from build123d import *

# Parameters (mm, degrees)
SKETCH2_W           = 21
SKETCH2_H           = 21
BOSS_EXTRUDE1_DEPTH = 20
SKETCH3_W           = 15
SKETCH3_H           = 15
CUT_EXTRUDE1_DEPTH  = 20
SKETCH4_W           = 4
SKETCH4_H           = 7.5
BOSS_EXTRUDE2_DEPTH = 20
FILLET2_R           = 2
SKETCH5_W           = 7
SKETCH5_H           = 56
BOSS_EXTRUDE3_DEPTH = 4
SKETCH6_W           = 3
SKETCH6_H           = 56
BOSS_EXTRUDE4_DEPTH = 85
SKETCH8_R           = 1.375
CUT_EXTRUDE2_DEPTH  = 4


with BuildPart() as part:
    # Sketch2 → Boss-Extrude1 (new body)
    with BuildSketch(Plane.XY):
        Rectangle(SKETCH2_W, SKETCH2_H)
    extrude(amount=BOSS_EXTRUDE1_DEPTH)

    # Sketch3 → Cut-Extrude1 (cut)
    with BuildSketch(Plane.XY.offset(20)):
        Rectangle(SKETCH3_W, SKETCH3_H)
    extrude(amount=-CUT_EXTRUDE1_DEPTH, mode=Mode.SUBTRACT)

    # Sketch4 → Boss-Extrude2 (add)
    with BuildSketch(Plane.ZY.offset(10.5)):
        with Locations((2, 0)):
            Rectangle(SKETCH4_W, SKETCH4_H)
    extrude(amount=BOSS_EXTRUDE2_DEPTH)

    # Fillet2
    fillet2_edges = [part.edges().sort_by_distance(p)[0] for p in [
        (-20.5, -3.75, 4),
        (-20.5, 3.75, 4),
    ]]
    fillet(fillet2_edges, radius=FILLET2_R)

    # Sketch5 → Boss-Extrude3 (add)
    with BuildSketch(Plane.ZY.offset(30.5)):
        with Locations((3.5, 0)):
            Rectangle(SKETCH5_W, SKETCH5_H)
    extrude(amount=BOSS_EXTRUDE3_DEPTH)

    # Sketch6 → Boss-Extrude4 (add)
    with BuildSketch(Plane.ZY.offset(34.5)):
        with Locations((1.5, 0)):
            Rectangle(SKETCH6_W, SKETCH6_H)
    extrude(amount=BOSS_EXTRUDE4_DEPTH)

    # Sketch8 → Cut-Extrude2 (cut)
    with BuildSketch(Plane.XY.offset(3)):
        with Locations((-39, -24.5)):
            Circle(SKETCH8_R)
        with Locations((-39, 24.5)):
            Circle(SKETCH8_R)
        with Locations((-97, -24.5)):
            Circle(SKETCH8_R)
        with Locations((-97, 24.5)):
            Circle(SKETCH8_R)
    extrude(amount=-CUT_EXTRUDE2_DEPTH, mode=Mode.SUBTRACT)


solid = part.part
Geometry: final body of the model. Coordinates: model frame, mm. A direction names the side the tool comes from. Coordinates: 2 decimals unless noted, no trailing zeros. Order: outer loops, then holes, each group sorted by start corner. A loop starts at its lowest first (then second) coordinate and runs counter-clockwise, first axis right, second up.
(1) Draft query along X for faces 1 (the face through (0, -10.5, 10)), 2 (the face through (-119.5, 0, 1)), 3 (the face through (-40.013, 25.429, 1.521)). Return one class per face: pulls with the +X half, pulls with the -X half, needs draft (parallel to the pull), parting line crosses it, or undercut.
(2) Section query D-D (x = -25). Return the cut outline in (y, z).
(3) Section query C-C (y = 15.5). Return the cut outline in (x, z), plus the area to 3 significant figures.
(4) First-contact query: pin 1 (4.5 mm diameter, centred on x = 1.5, z = 5.5, fed in from -Y); pin 2 (3 mm diameter, centred on x = -37.5, z = 7.5, fed in from +Y); pin 3 (8 mm diameter, centred on y = 14, z = 13.5, fed in from -X); pin 4 (3 mm diameter, centred on y = 1.5, z = 5.5, fed in from -X). Flat tips, straight axial feed; report the tip coordinate or a pass-through.
(5) Access query for faces 4 (the face through (-20, 0, 4)), 5 (the face through (0, 7.5, 10)), 6 (the face through (-32, 0, 7)), 7 (the face through (0, 10.5, 10)). Directions: +Z, -Z, +X, -X, +Y, -Y. A direction counts if a zero-diameter tool reaches every point of the face in a straight line with its end or side. Return the directions, or none.
(6) Section query B-B (y = -24.5). Return the cut outline in (x, z) (3 decimals).
(7) Material intervals for probe 1 along X at (y, z) = (-3, 6.5); probe 2 along X at (y, z) = (-6.5, 2.5); probe 3 along Y at (x, z) = (-97, 1.7) (3 decimals), sorted ascending.
(8) Section query A-A (x = -97). Return the cut outline in (y, z) (3 decimals), plus the area to 4 significant figures.
Solution:
1. face 1: needs draft
1. face 2: pulls with the -X half
1. face 3: undercut
2. outline: (-3.75, 0) - (3.75, 0) - (3.75, 2) arc R2 ccw to (1.75, 4) - (-1.75, 4) arc R2 ccw to (-3.75, 2) - close
3. outline: (-119.5, 0) - (-30.5, 0) - (-30.5, 7) - (-34.5, 7) - (-34.5, 3) - (-119.5, 3) - close
3. area: 283 mm2
4. pin 1: stops at y = -10.5
4. pin 2: passes through
4. pin 3: stops at x = -10.5
4. pin 4: stops at x = -34.5
5. face 4: +Z, +Y, -Y
5. face 5: +Z, -Z
5. face 6: +Z, -X, +Y, -Y
5. face 7: +Z, -Z, +X, +Y
6. outline: (-119.5, 0) - (-98.375, 0) - (-98.375, 3) - (-119.5, 3) - close; (-95.625, 0) - (-40.375, 0) - (-40.375, 3) - (-95.625, 3) - close; (-37.625, 0) - (-30.5, 0) - (-30.5, 7) - (-34.5, 7) - (-34.5, 3) - (-37.625, 3) - close
7. probe 1: x = -34.5 to -30.5, -10.5 to -7.5, 7.5 to 10.5
7. probe 2: x = -119.5 to -30.5, -10.5 to -7.5, 7.5 to 10.5
7. probe 3: y = -28 to -25.875, -23.125 to 23.125, 25.875 to 28
8. outline: (-28, 0) - (-25.875, 0) - (-25.875, 3) - (-28, 3) - close; (-23.125, 0) - (23.125, 0) - (23.125, 3) - (-23.125, 3) - close; (25.875, 0) - (28, 0) - (28, 3) - (25.875, 3) - close
8. area: 151.5 mm2
